Here's the drawing with two shaded views (mm, measured from the low corner). I have some questions. A direction names the side the tool comes from. Coordinates: 2 decimals unless noted, no trailing zeros. Write each loop counter-clockwise with the first axis right and the second up, starting at its lowest first coordinate (ties: lowest second). Pieces come first, ordered by that corner, then holes. Notation, with made-up numbers: (9.25, 48.25) - (16.25, 48.25) arc R12 ccw to (16.25, 55.25) - close; hole circle Ø2 at (65, 77.5). An arc over 180 degrees is marked (long way). Answer in a Markdown table with one row per item. Add a question column.
Item 1: Imagine slicing it at C-C (x = 5.75). Please give me the cut outline in (y, z), plus the area to 3 significant figures.
Item 2: We'd pull the mould along Z, two halves only. Please class the marked faces 4, 5 and 6: +Z half, -Z half, draft (parallel to the pull), parting line (faces both ways), or undercut.
Item 3: Which directions (+Z, -Z, +X, -X, +Y, -Y) give clear straight access to the entire face, cutting with the end or side of a thin tool? Please do the marked faces 1, 2 and 3.
Item 4: If I drill on probe 1 along Z at (x, y) = (11, 3.5); probe 2 along Y at (x, z) = (16.25, 18.5); probe 3 along X at (y, z) = (4.25, 9), over which ranges is the centre line in solid material (lowest first)? Write a range as from..to.
Item 5: Imagine slicing it at D-D (y = 5). Please give me the cut outline in (x, z).
Item 6: Imagine slicing it at B-B (z = 6.25). Please give me the cut outline in (x, y).
Item 7: Imagine slicing it at A-A (x = 11). Please give me the cut outline in (y, z).
Item 8: I'm going to push flat-ended pins straight in: pin 1 (2 mm diameter, centred on y = 3.5, z = 9.5, fed in from -X); pin 2 (4 mm diameter, centred on y = 6.5, z = 6.5, fed in from -X); pin 3 (1 mm diameter, centred on y = 3, z = 10, fed in from +X). Where does each tip first touch, or does it pass through?
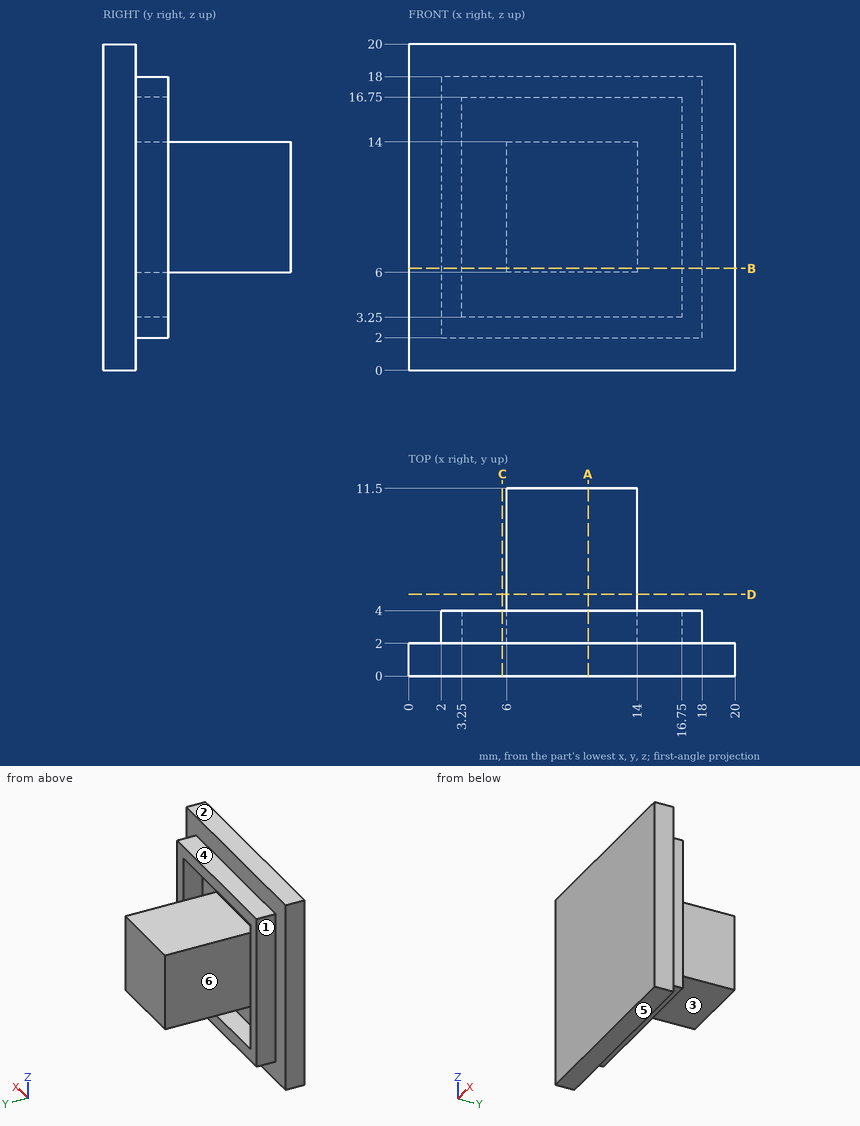
Here are the results:
| question | item | result |
|---|---|---|
| 1 | outline | (0, 0) - (2, 0) - (2, 2) - (4, 2) - (4, 3.25) - (2, 3.25) - (2, 16.75) - (4, 16.75) - (4, 18) - (2, 18) - (2, 20) - (0, 20) - close |
| 1 | area | 45.0 mm2 |
| 2 | face 4 | +Z half |
| 2 | face 5 | -Z half |
| 2 | face 6 | undercut |
| 3 | face 1 | +Z, -Z, -X, +Y |
| 3 | face 2 | +Z, +X, -X, +Y, -Y |
| 3 | face 3 | +Y |
| 4 | probe 1 | z = 2..3.25, 6..14, 16.75..18 |
| 4 | probe 2 | y = 0..2 |
| 4 | probe 3 | x = 6..14 |
| 5 | outline | (6, 6) - (14, 6) - (14, 14) - (6, 14) - close |
| 6 | outline | (0, 0) - (20, 0) - (20, 2) - (18, 2) - (18, 4) - (16.75, 4) - (16.75, 2) - (14, 2) - (14, 11.5) - (6, 11.5) - (6, 2) - (3.25, 2) - (3.25, 4) - (2, 4) - (2, 2) - (0, 2) - close |
| 7 | outline | (0, 0) - (2, 0) - (2, 2) - (4, 2) - (4, 3.25) - (2, 3.25) - (2, 6) - (11.5, 6) - (11.5, 14) - (2, 14) - (2, 16.75) - (4, 16.75) - (4, 18) - (2, 18) - (2, 20) - (0, 20) - close |
| 8 | pin 1 | stops at x = 2 |
| 8 | pin 2 | stops at x = 6 |
| 8 | pin 3 | stops at x = 18 |
